The drawing under review shows one solid part. Ordinate dimensions are in mm from its lowest x, y, z. A direction names the side the tool comes from. Round coordinates to 2 decimals unless told otherwise and drop trailing zeros. Order: outer loops, then holes, each group sorted by start corner. A loop starts at its lowest first (then second) coordinate and runs counter-clockwise, first axis right, second up.
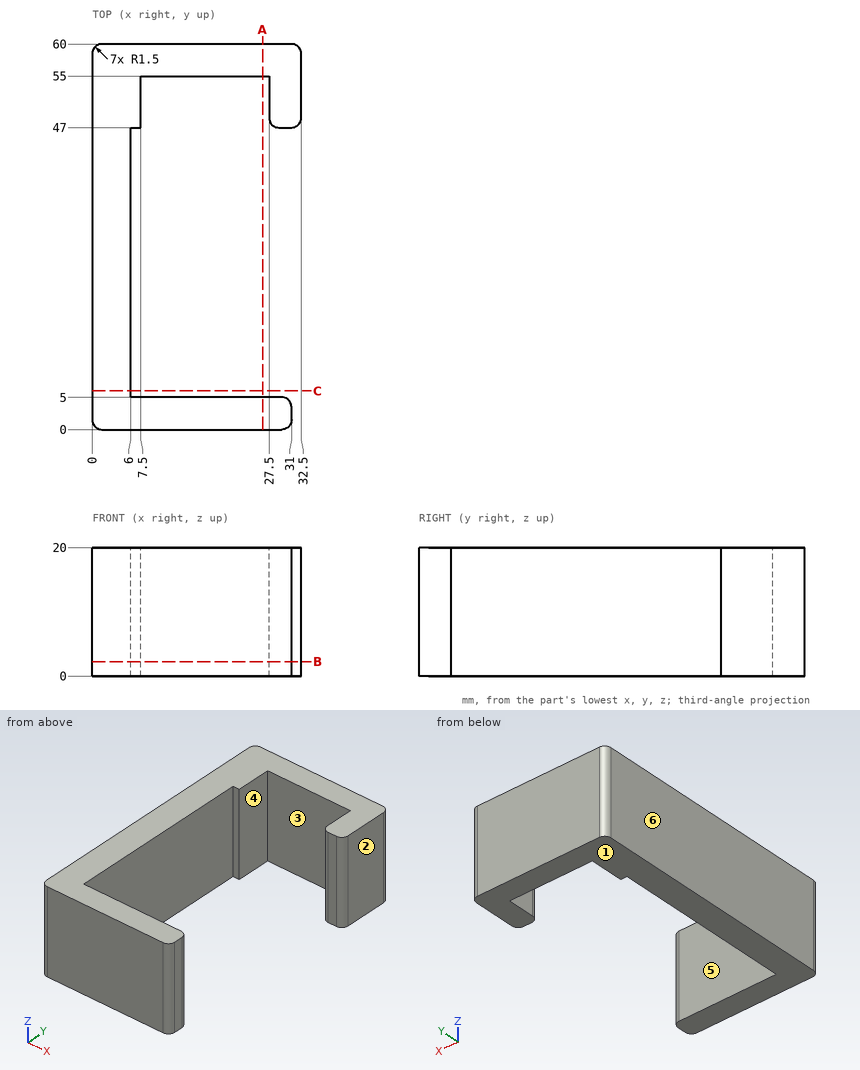
(1) Clearance check with flat-ended pins moving along their axes: P1, Ø5, axis at y = 28.5, z = 4.5, coming from the +X side; P2, Ø2, axis at y = 2.5, z = 14, coming from the +X side. State where each tip first meets the part, or that it passes through.
(2) The part is to be moulded in two halves that separate along X. For the marked faces 1, 2, 3 and 4, say which applies: pulls with the +X half, pulls with the -X half, needs draft (parallel to the pull), parting line crosses it, or undercut.
(3) To check wall thickness, follow L1, parallel to Y at x = 19.5, z = 6.5; L2, parallel to X at y = 52, z = 17; L3, parallel to Y at x = 29, z = 3.5. State the ranges of each line that lie inside material, in increasing order.
(4) We need section B-B (z = 2.25). Give the boundary of the cut face in (x, y), and give its area (3 significant figures).
(5) We need section C-C (y = 6). Give the boundary of the cut face in (x, z).
(6) We need section A-A (x = 26.5). Give the boundary of the cut face in (y, z).
(7) Tool access review of the marked faces 5 and 6: name each direction out of +Z, -Z, +X, -X, +Y, -Y from which nothing blocks a thin tool from reaching the whole face with its end or side.
Verdict:
1. P1: stops at x = 6
1. P2: stops at x = 31
2. face 1: needs draft
2. face 2: pulls with the +X half
2. face 3: undercut
2. face 4: undercut
3. L1: y = 0 to 5, 55 to 60
3. L2: x = 0 to 7.5, 27.5 to 32.5
3. L3: y = 0 to 5, 47 to 60
4. outline: (0, 1.5) arc R1.5 ccw to (1.5, 0) - (29.5, 0) arc R1.5 ccw to (31, 1.5) - (31, 3.5) arc R1.5 ccw to (29.5, 5) - (6, 5) - (6, 47) - (7.5, 47) - (7.5, 55) - (27.5, 55) - (27.5, 48.5) arc R1.5 ccw to (29, 47) - (31, 47) arc R1.5 ccw to (32.5, 48.5) - (32.5, 58.5) arc R1.5 ccw to (31, 60) - (1.5, 60) arc R1.5 ccw to (0, 58.5) - close
4. area: 666 mm2
5. outline: (0, 0) - (6, 0) - (6, 20) - (0, 20) - close
6. outline: (0, 0) - (5, 0) - (5, 20) - (0, 20) - close; (55, 0) - (60, 0) - (60, 20) - (55, 20) - close
7. face 5: +Z, -Z, +X
7. face 6: +Z, -Z, -X, +Y, -Y
